Geometry check sheet. Reference: the model listing, model coordinates, mm. A direction names the side the tool comes from. Round coordinates to 2 decimals unless told otherwise and drop trailing zeros. Loops run counter-clockwise (first coordinate to the right, second up) from the corner with the lowest first, then second, coordinate; pieces in that order, holes last. Notation, with made-up numbers: (-4, 9.25) - (10, 9.25) arc R22 cw to (10, 29.25) - close; hole circle Ø3 at (50.25, -27). An arc over 180 degrees is marked (long way). Answer as CSV lines item,"result". Start each with the question number.
1) Draft check along X on faces 1 (the flat face through (1, 115, 2)), 2 (the cylindrical face through (-8, -76, 2)), 3 (the flat face through (90, -1, 2)). Enter one of: released by +X, released by -X, zero draft, split by the parting line, or undercut.
2) Access from +Z, -Z, +X, -X, +Y, -Y to the whole of each face (thin tool, end or side, straight path). Record for faces 4 (the cylindrical face through (9, -77, 2)), 5 (the cylindrical face through (-84.297, -108.986, 2.218)).
3) Thickness scan on line 1 along X through (y, z) = (-86, 1.25); line 2 along Y through (x, z) = (-71, 0.5); line 3 along X through (y, z) = (95.5, 3.45). Record the ranges inside material, lowest first.
4) Cross-section at B-B on x = 79. Record the boundary of the cut face in (y, z).
5) Cross-section at A-A on z = 3.15. Record the boundary of the cut face in (x, y), and give its area (3 significant figures).
6) Depth check by flat-ended pin: P1, Ø1.3, axis at y = -102.5, z = 1.5, coming from the +X side; P2, Ø2, axis at y = -99.5, z = 1, coming from the -X side. Enter the tip coordinate at first touch or a pass-through.
from build123d import *

# Parameters (mm, degrees)
EXTRUDE_1_DEPTH     = 4.5
CUT_EXTRUDE_1_DEPTH = 4.5


with BuildPart() as part:
    # 草图1 → 凸台-拉伸1 (new body)
    with BuildSketch(Plane.XY):
        with BuildLine():
            Line((-70, -115), (70, -115))
            ThreePointArc((70, -115), (84.142135624, -109.142135624), (90, -95))
            Line((90, -95), (90, 95))
            ThreePointArc((90, 95), (84.142135624, 109.142135624), (70, 115))
            Line((70, 115), (-70, 115))
            ThreePointArc((-70, 115), (-84.142135624, 109.142135624), (-90, 95))
            Line((-90, 95), (-90, -95))
            ThreePointArc((-90, -95), (-84.142135624, -109.142135624), (-70, -115))
        make_face()
    extrude(amount=EXTRUDE_1_DEPTH)

    # 草图2 → 切除-拉伸1 (cut)
    with BuildSketch(Plane.XY.offset(4.5)):
        with BuildLine():
            Line((-10, -155), (10, -155))
            Line((10, -155), (10, -80))
            ThreePointArc((10, -80), (8.535533906, -76.464466094), (5, -75))
            Line((5, -75), (-5, -75))
            ThreePointArc((-5, -75), (-8.535533906, -76.464466094), (-10, -80))
            Line((-10, -80), (-10, -155))
        make_face()
    extrude(amount=-CUT_EXTRUDE_1_DEPTH, mode=Mode.SUBTRACT)


solid = part.part
Answer block:
1,face 1,"zero draft"
1,face 2,"undercut"
1,face 3,"released by +X"
2,face 4,"+Z, -Z, -Y"
2,face 5,"+Z, -Z, -X, -Y"
3,line 1,"x = -90 to -10, 10 to 90"
3,line 2,"y = -114.97 to 114.97"
3,line 3,"x = -89.99 to 89.99"
4,outline,"(-112.86, 0) - (112.86, 0) - (112.86, 4.5) - (-112.86, 4.5) - close"
5,outline,"(-90, -95) arc R20 ccw to (-70, -115) - (-10, -115) - (-10, -80) arc R5 cw to (-5, -75) - (5, -75) arc R5 cw to (10, -80) - (10, -115) - (70, -115) arc R20 ccw to (90, -95) - (90, 95) arc R20 ccw to (70, 115) - (-70, 115) arc R20 ccw to (-90, 95) - close"
5,area,"40,300 mm^2"
6,P1,"stops at x = 88.79"
6,P2,"stops at x = -89.69"
